Here's how the part is built. I have some questions about the finished solid (model axes, mm). Give positions to 0.01 mm unless a question says otherwise; leave off trailing zeros. Order: outer loops, then holes, each group sorted by start corner. A loop starts at its lowest first (then second) coordinate and runs counter-clockwise, first axis right, second up.
from build123d import *

# Parameters (mm, degrees)
F14_DEPTH = 1


with BuildPart() as f14:
    # F13 (on offset) → F14 (new body)
    with BuildSketch(Plane.XY.offset(-76)):
        Polygon((0, -751.526058), (0, 0), (-3.126378, -49.995076), (-3.126378, -747.989655), align=None)
    extrude(amount=-F14_DEPTH)

    # F15: F14 across face


with BuildPart() as f14_1:
    add(f14.part)
    add(f14.part.mirror(Plane(origin=(0, -375.763029, -76.5), x_dir=(0, 1, 0), z_dir=(1, 0, 0))))


solid = f14_1.part
Q1. If we section it at A-A on z = -76.25: List the corners of the cut face in (x, y) for me, plus the area to 3 significant figures.
Filled sheet:
outline: (-3.13, -747.99) - (0, -751.53) - (3.13, -747.99) - (3.13, -50) - (0, 0) - (-3.13, -50) - close
area: 4,530 mm2
Q2. I need wall thicknesses on L1, parallel to X at y = -43, z = -76.55. Which ranges of the line are inside material? Lowest first, please.
Filled sheet:
L1: x = -2.69 to 2.69
Q3. If we section it at B-B on x = 1.75: List the corners of the cut face in (y, z) for me, plus the area to 3 significant figures.
Filled sheet:
outline: (-749.55, -77) - (-27.98, -77) - (-27.98, -76) - (-749.55, -76) - close
area: 722 mm2
